Geometry check sheet. Reference: drawing and pictorial views, mm from the part's lowest x, y, z. A direction names the side the tool comes from. Give positions to 0.01 mm unless a question says otherwise; leave off trailing zeros. Write each loop counter-clockwise with the first axis right and the second up, starting at its lowest first coordinate (ties: lowest second). Pieces come first, ordered by that corner, then holes. Notation, with made-up numbers: M 21.5,-8.5 L 29.5,-8.5 A13 ccw 29.5,-2.5 Z; hole C 13,11.25 d1. An arc over 180 degrees is marked long. Answer as a JSON object with one key per item and string values.
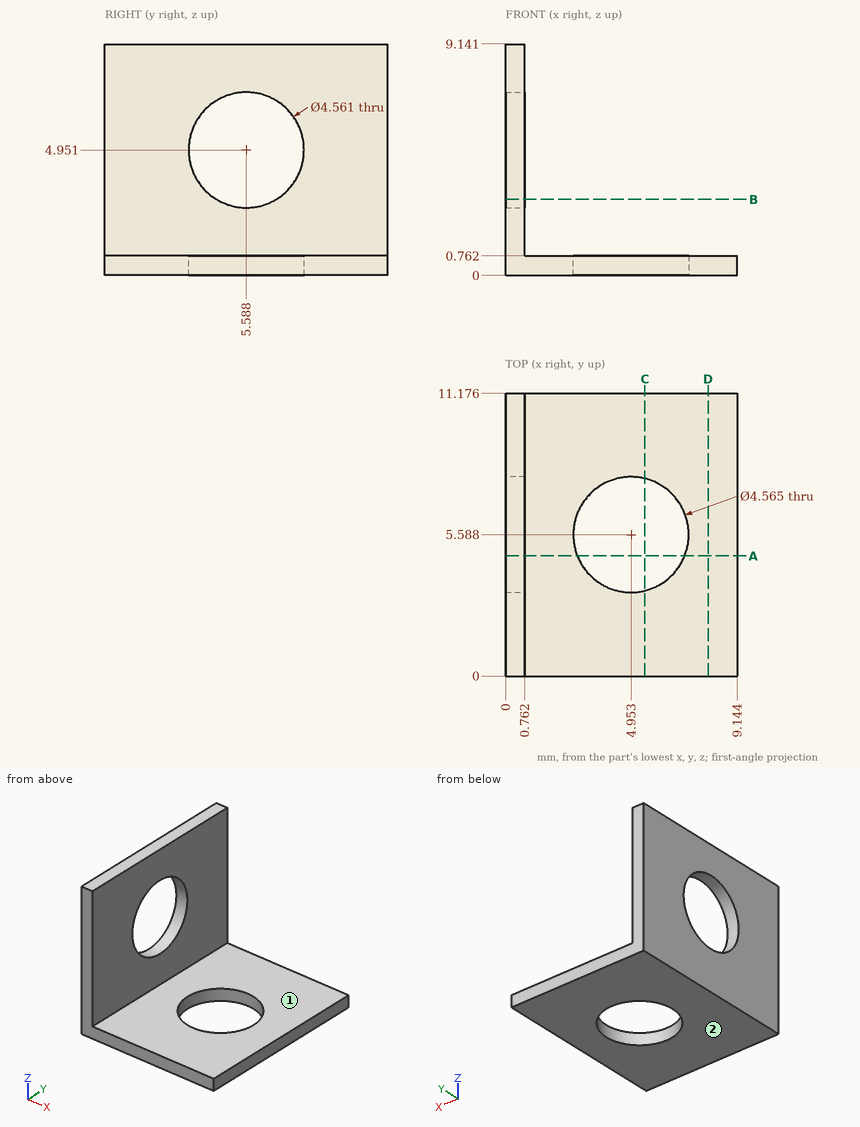
1) Section check B-B on z = 3. Record the boundary of the cut face in (x, y).
Completed:
{"outline": "M 0,0 L 0.76,0 L 0.76,4.41 L 0,4.41 Z; M 0,6.77 L 0.76,6.77 L 0.76,11.18 L 0,11.18 Z"}
2) Section check D-D on x = 8. Record the boundary of the cut face in (y, z).
Completed:
{"outline": "M 0,0 L 11.18,0 L 11.18,0.76 L 0,0.76 Z"}
3) Thickness scan on L1, parallel to Z at x = 1, y = 9. Record the ranges inside material, lowest first.
Completed:
{"L1": "z = 0 to 0.76"}
4) Go/stop test with flat-tipped pins: pin 1 (2.5 mm diameter, centred on x = 5, y = 3.5, fed in from +Z); pin 2 (1.5 mm diameter, centred on y = 6, z = 7.5, fed in from +X); pin 3 (2.5 mm diameter, centred on x = 4.95, y = 5.59, fed in from -Z) (3 decimals); pin 4 (3 mm diameter, centred on y = 5.5, z = 1, fed in from +X). Record where each tip stops, or that it passes through.
Completed:
{"pin 1": "stops at z = 0.76", "pin 2": "stops at x = 0.76", "pin 3": "passes through", "pin 4": "stops at x = 9.14"}
5) Access from +Z, -Z, +X, -X, +Y, -Y to the whole of each face (thin tool, end or side, straight path). Record for the marked faces 1 and 2.
Completed:
{"face 1": "+Z, +X, +Y, -Y", "face 2": "-Z, +X, -X, +Y, -Y"}
6) Section check C-C on x = 5.5. Record the boundary of the cut face in (y, z).
Completed:
{"outline": "M 0,0 L 3.37,0 L 3.37,0.76 L 0,0.76 Z; M 7.8,0 L 11.18,0 L 11.18,0.76 L 7.8,0.76 Z"}
7) Section check A-A on y = 4.75. Record the boundary of the cut face in (x, z) (1 decimal).
Completed:
{"outline": "M 0,0 L 2.8,0 L 2.8,0.8 L 0.8,0.8 L 0.8,2.8 L 0,2.8 Z; M 0,7.1 L 0.8,7.1 L 0.8,9.1 L 0,9.1 Z; M 7.1,0 L 9.1,0 L 9.1,0.8 L 7.1,0.8 Z"}
